Work out the finished part from the listing and answer in its coordinate system (mm). A direction names the side the tool comes from. Give positions to 0.01 mm unless a question says otherwise; leave off trailing zeros. Loops run counter-clockwise (first coordinate to the right, second up) from the corner with the lowest first, then second, coordinate; pieces in that order, holes last. Notation, with made-up numbers: (22.25, -27) - (63.25, -27) arc R14 ccw to (63.25, -19) - close; hole circle Ø5 at (22.25, -21.75). An arc over 180 degrees is marked (long way). Use CSV: the item, a comma, the result in double quotes.
Autodesk Inventor part; units mm, degrees
ref_plane "YZ Plane" through (0, 0, 0) normal (1, 0, 0) x (0, 1, 0)
ref_plane "XZ Plane" through (0, 0, 0) normal (0, 1, 0) x (-1, 0, 0)
ref_plane "XY Plane" through (0, 0, 0) normal (0, 0, 1) x (1, 0, 0)
sketch "Sketch1 outline for Plate1" plane through (0, 0, 0) normal (0, 0, 1) x (1, 0, 0)
  line L0 (53.975, 44.45) -> (53.975, 19.05)
  line L1 (53.975, 19.05) -> (53.975, -25.4)
  line L2 (53.975, -25.4) -> (22.225, -25.4)
  line L3 (22.225, -25.4) -> (22.225, -59.055)
  line L4 (22.225, -59.055) -> (0, -59.055)
  line L5 (0, -59.055) -> (0, 0)
  line L6 (0, 0) -> (22.225, 0)
  line L7 (22.225, 0) -> (22.225, 50.8)
  line L8 (22.225, 50.8) -> (47.625, 50.8)
  line L9 (47.625, 50.8) -> (53.975, 50.8)
  line L10 (53.975, 50.8) -> (53.975, 44.45)
extrude "Plate1" add sketch "Sketch1 outline for Plate1" along normal blind 3.175
sketch "Sketch2" plane through (0, -55.88, 3.175) normal (0, -1, 0) x (1, 0, 0)
  line L0 (22.225, 0) -> (0, 0)
  line L1 (0, 0) -> (0, -31.75)
  line L2 (0, -31.75) -> (22.225, -31.75)
  line L3 (22.225, -31.75) -> (22.225, 0)
edge flange "Flange1" height 31.75 angle 90 thickness 3.175 bend radius 3.175 thickness toward (0, -1, 0) relief straight relief width 3.175 relief depth 1.5875 edges at (11.1125, -59.055, 0) wall of the first edge with corners at (22.225, -55.88, 3.175) (0, -55.88, 3.175) (0, -55.88, -28.575) (22.225, -55.88, -28.575)
bend "Bend1"
corner "Corner1"
sketch "Sketch3" plane through (0, -55.88, -28.575) normal (0, 1, 0) x (1, 0, 0)
  circle A0 centre (12.7, -12.7) radius 3.3782
  point P0 (0, -28.575)
extrude "Cut1" cut sketch "Sketch3" against normal blind 3.175
sketch "Sketch1" plane through (0, 0, 0) normal (0, 0, 1) x (1, 0, 0)
  line L0 (0, 0) -> (82.111681, 0)
  line L1 (56.711681, -22.225) -> (0, -22.225)
  line L2 (85.286681, -3.175) -> (85.286681, -19.05)
  line L3 (29.00734, 0) -> (29.00734, -1.5875)
  line L4 (29.00734, -1.5875) -> (28.21359, -1.5875)
  line L5 (29.00734, -1.5875) -> (29.80109, -1.5875)
  line L6 (29.80109, -1.5875) -> (29.80109, 0)
  line L7 (28.21359, -1.5875) -> (28.21359, 0)
  line L8 (29.80109, -22.225) -> (29.80109, -20.6375)
  line L9 (29.80109, -20.6375) -> (28.21359, -20.6375)
  line L10 (28.21359, -20.6375) -> (28.21359, -22.225)
sketch "Sketch5" plane through (53.975, -25.4, 0) normal (1, 0, 0) x (0, 0, -1)
  line L0 (-3.175, 76.2) -> (-3.175, 0)
  line L1 (0, 76.2) -> (0, 0)
  line L2 (0, 76.2) -> (-3.175, 76.2)
  line L3 (-3.175, 76.2) -> (-3.175, 38.1)
  line L4 (-3.175, 38.1) -> (0, 38.1)
  point P0 (0, 25.4)
  dimension "d13" = 38.1
extrude "Extrusion1" add sketch "Sketch5" along normal blind 38.1
sketch "Sketch6" plane through (22.225, 50.8, 3.175) normal (0, 1, 0) x (1, 0, 0)
  line L0 (0, 0) -> (69.85, 0)
  line L1 (69.85, 3.175) -> (69.85, 0)
  line L2 (0, 3.175) -> (69.85, 3.175)
  line L3 (0, 3.175) -> (0, 0)
  point P0 (-22.225, 3.175)
extrude "Extrusion2" add sketch "Sketch6" along normal blind 12.7
fillet "Fillet2" radius 3.175 8 edges at (22.225, 63.5, 1.5875) (92.075, 63.5, 1.5875) (22.225, 0, 1.5875) (0, 0, 1.5875) (92.075, 12.7, 1.5875) (53.975, 12.7, 1.5875) (53.975, -25.4, 1.5875) (22.225, -25.4, 1.5875)
equation "\"d1\" = BendReliefWidth"
equation "\"d2\" = BendReliefDepth"
equation "\"d3\" = MinimumRemnant"
equation "\"d4\" = BendRadius"
equation "\"d7\" = BendRadius"
equation "\"d8\" = CornerReliefSize"
equation "\"d9\" = GapSize"
equation "\"d10\" = JacobiRadiusSize"
equation "\"BendRadius\" = Thickness"
equation "\"BendReliefWidth\" = Thickness"
equation "\"BendReliefDepth\" = 0.5 * Thickness"
equation "\"CornerReliefSize\" = 4 * Thickness"
equation "\"MinimumRemnant\" = 2 * Thickness"
equation "\"TransitionRadius\" = BendRadius"
equation "\"JacobiRadiusSize\" = Thickness"
equation "\"GapSize\" = Thickness"
equation "\"d0\" = BendRadius"
equation "\"d4\" = Thickness"
properties part number "cylinder mount" material "Aluminum 6061"
Item 1: For faces 1 (the flat face through (73, 12.7, 2)), 2 (the flat face through (45, 17, 3.175)), 3 (the flat face through (11, 0, 2)), 4 (the flat face through (0, -39.5, 0.2)), 5 (the flat face through (8, -55.88, -16)), determine the directions among +Z, -Z, +X, -X, +Y, -Y from which every point of the face is accessible in a straight line to the end or side of a thin tool.
Determined:
face 1,"+Z, -Z, +X, -Y"
face 2,"+Z, +X, -X, +Y, -Y"
face 3,"+Z, -Z, -X, +Y"
face 4,"+Z, -Z, -X, +Y, -Y"
face 5,"-Z, +X, -X, +Y"
Item 2: Given P1, Ø5, axis at x = 18.5, y = 40.5, coming from the -Z side; P2, Ø8, axis at x = 12.7, z = -15.875, coming from the -Y side (3 decimals); P3, Ø2.5, axis at x = 8, z = 2, coming from the +Y side; P4, Ø18, axis at x = 7.5, z = -19, coming from the +Y side, each flat-ended and moving along its own axis, determine where each tip first touches the part or whether it passes through.
Determined:
P1,"passes through"
P2,"stops at y = -59.055"
P3,"stops at y = 0"
P4,"stops at y = -55.88"
Item 3: Find the intervals of material crossed by line 1 (Z direction, x = 7, y = -17.5) (3 decimals); line 2 (Y direction, x = 9.5, z = -24) (3 decimals); line 3 (Z direction, x = 12.7, y = -56.95) (3 decimals), in increasing order.
Determined:
line 1,"z = 0 to 3.175"
line 2,"y = -59.055 to -55.88"
line 3,"z = -28.575 to -19.253, -12.497 to 1.548"
Item 4: A cutting plane is placed at A-A on x = 12.7. Determine the outline of the cut face in (y, z) (3 decimals), and give its area (3 significant figures).
Determined:
outline,"(-59.055, -28.575) - (-55.88, -28.575) - (-55.88, -19.253) - (-59.055, -19.253) - close; (-59.055, -12.497) - (-55.88, -12.497) - (-55.88, -3.175) arc R3.175 cw to (-52.705, 0) - (0, 0) - (0, 3.175) - (-52.705, 3.175) arc R6.35 ccw to (-59.055, -3.175) - close"
area,"250 mm²"
Item 5: A cutting plane is placed at B-B on y = -35.5. Determine the outline of the cut face in (x, z) (3 decimals), and give its area (3 significant figures).
Determined:
outline,"(0, 0) - (22.225, 0) - (22.225, 3.175) - (0, 3.175) - close"
area,"70.6 mm²"
Item 6: A cutting plane is placed at C-C on x = 46. Determine the outline of the cut face in (y, z) (3 decimals).
Determined:
outline,"(-25.4, 0) - (63.5, 0) - (63.5, 3.175) - (-25.4, 3.175) - close"
